Model file for the job. Use its own axes, mm. Face numbers are marked on the shaded views. A direction names the side the tool comes from. Round coordinates to 2 decimals unless told otherwise and drop trailing zeros. Order: outer loops, then holes, each group sorted by start corner. A loop starts at its lowest first (then second) coordinate and runs counter-clockwise, first axis right, second up. Notation, with made-up numbers: M -38,-26.5 L -33,-26.5 A27 cw -33,-8.5 Z; hole C 18.5,62.25 d1. An arc over 180 degrees is marked long. Return JSON: item names as keys, results as strings. Group by question number.
Item 1: Slice it at D-D on z = -21.25. Write the cut outline in (x, y), then the cut area to 3 significant figures.
Item 2: Pin check, flat tips, straight feed: pin 1 Ø1.8 at (x, z) = (-50, -23) entering from +Y; pin 2 Ø2 at (x, y) = (-49.5, 8.5) entering from +Z; pin 3 Ø0.6 at (x, y) = (-60, 6.5) entering from +Z. Stop position of each tip, or through.
Item 3: Which spindle directions (+Z, -Z, +X, -X, +Y, -Y) get a long thin tool onto all of the face, cutting with end or side? Do the marked faces 4, 5 and 6. Say none if no direction does.
Item 4: Slice it at A-A on y = 2.25. Write the cut outline in (x, z).
Item 5: Pull direction X, two halves, no side cores. Call the marked faces 1, 2 and 3: pulls with the +X half, pulls with the -X half, needs draft (parallel to the pull), parting line crosses it, or undercut.
Item 6: Probe line 1 along X through (y, z) = (3.75, -32.5); line 2 along Z through (x, y) = (-60, 3); line 3 along Y through (x, z) = (-51, -21.75). List the from-to ranges inside material, lowest first.
Item 7: Slice it at C-C on x = -44. Write the cut outline in (y, z), then the cut area to 4 significant figures.
Item 8: Slice it at B-B on y = 6.75. Write the cut outline in (x, z), then the cut area to 3 significant figures.
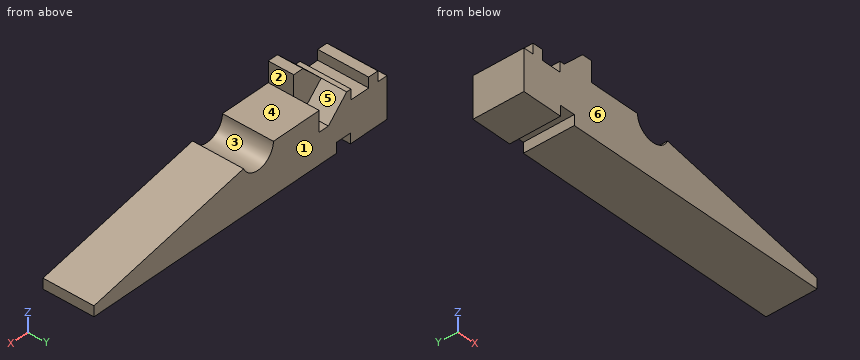
from build123d import *

# Parameters (mm, degrees)
PAD_DEPTH       = 10
SKETCH001_R     = 3.4
POCKET_DEPTH    = 10.001
PAD001_DEPTH    = 5
POCKET001_DEPTH = 5


with BuildPart() as part:
    # Sketch → Pad (new body)
    with BuildSketch(Plane(origin=(0, 0, 0), x_dir=(1, 0, 0), z_dir=(0, 1, 0))):
        Polygon((-62.846755, 25.248808), (-60.846755, 25.248808), (-60.846755, 23.248808), (-58.846755, 23.248808), (-58.846755, 25.248808), (-54.972908, 25.248808), (-54.972908, 23.248808), (-38.042093, 23.248808), (1.153245, 31.231634), (1.153245, 33.248808), (-51.846755, 33.248808), (-51.846755, 31.248808), (-54.846755, 31.248808), (-54.846755, 33.248808), (-62.846755, 33.248808), align=None)
    extrude(amount=PAD_DEPTH)

    # Sketch001 → Pocket (cut, through all)
    with BuildSketch(Plane(origin=(0, 10, 0), x_dir=(1, 0, 0), z_dir=(0, 1, 0))):
        with Locations((-34.642093, 23.248808)):
            Circle(SKETCH001_R)
    extrude(amount=-POCKET_DEPTH, mode=Mode.SUBTRACT)

    # Sketch002 → Pad001 (new body)
    with BuildSketch(Plane.XZ):
        Polygon((-48.042093, -23.248808), (-48.042093, -19.248808), (-50.042093, -19.248808), (-54.042093, -23.248808), align=None)
    extrude(amount=-PAD001_DEPTH)

    # Sketch003 → Pocket001 (cut)
    with BuildSketch(Plane(origin=(0, 10, 0), x_dir=(1, 0, 0), z_dir=(0, 1, 0))):
        Polygon((-48.042093, 23.248808), (-48.042093, 27.248808), (-50.042093, 27.248808), (-54.042093, 23.248808), align=None)
    extrude(amount=-POCKET001_DEPTH, mode=Mode.SUBTRACT)


solid = part.part
Output values:
{
 "1": {"outline": "M -52.04,0 L -48.04,0 L -48.04,5 L -52.04,5 Z", "area": "20.0 mm²"},
 "2": {"pin 1": "y = 5", "pin 2": "z = -26.79", "pin 3": "z = -23.25"},
 "3": {"face 4": "+Z, +X, +Y, -Y", "face 5": "+Z, +Y", "face 6": "+Z, -Z, +X, -X, -Y"},
 "4": {"outline": "M -62.85,-33.25 L -54.85,-33.25 L -54.85,-31.25 L -51.85,-31.25 L -51.85,-33.25 L 1.15,-33.25 L 1.15,-31.23 L -31.51,-24.58 A3.4 cw -38.04,-23.25 L -48.04,-23.25 L -48.04,-19.25 L -50.04,-19.25 L -54.04,-23.25 L -54.97,-23.25 L -54.97,-25.25 L -58.85,-25.25 L -58.85,-23.25 L -60.85,-23.25 L -60.85,-25.25 L -62.85,-25.25 Z"},
 "5": {"face 1": "needs draft", "face 2": "pulls with the +X half", "face 3": "undercut"},
 "6": {"line 1": "-62.85 to -54.85, -51.85 to 1.15", "line 2": "-33.25 to -23.25", "line 3": "0 to 5"},
 "7": {"outline": "M 0,-33.25 L 10,-33.25 L 10,-23.25 L 0,-23.25 Z", "area": "100.0 mm²"},
 "8": {"outline": "M -62.85,-33.25 L -54.85,-33.25 L -54.85,-31.25 L -51.85,-31.25 L -51.85,-33.25 L 1.15,-33.25 L 1.15,-31.23 L -31.51,-24.58 A3.4 cw -38.04,-23.25 L -48.04,-23.25 L -48.04,-27.25 L -50.04,-27.25 L -54.04,-23.25 L -54.97,-23.25 L -54.97,-25.25 L -58.85,-25.25 L -58.85,-23.25 L -60.85,-23.25 L -60.85,-25.25 L -62.85,-25.25 Z", "area": "436 mm²"}
}
